Read the model definition and answer for the solid it produces. Units are mm, in the model's axes. Coordinates: 2 decimals unless noted, no trailing zeros. Order: outer loops, then holes, each group sorted by start corner. A loop starts at its lowest first (then second) coordinate and runs counter-clockwise, first axis right, second up. Notation, with made-up numbers: (81.25, -25) -> (138.25, -25) arc R11 ccw to (138.25, -13) -> close; hole circle Ø9 at (89.5, 80.25). An arc over 180 degrees is marked (long way). Return JSON: item names as keys, results as strings. Group by question number.
```python
from build123d import *

# Parameters (mm, degrees)
IZIM1_R                     = 455
Y_KSEKLIK_EKSTR_ZYON1_DEPTH = 12
IZIM2_R                     = 12.5
KES_EKSTR_ZYON1_DEPTH       = 644.579054973
F_8_5_8_5_AP_DELIK1_D       = 8.5


with BuildPart() as part:
    # Çizim1 → Yükseklik-Ekstrüzyon1 (new body)
    with BuildSketch(Plane.XY):
        Circle(IZIM1_R)
    extrude(amount=Y_KSEKLIK_EKSTR_ZYON1_DEPTH)

    # Çizim2 → Kes-Ekstrüzyon1 (cut, through all)
    with BuildSketch(Plane.XY.offset(12)):
        Circle(IZIM2_R)
    extrude(amount=-KES_EKSTR_ZYON1_DEPTH, mode=Mode.SUBTRACT)

    # Ø8.5 (8.5) Çap Delik1 (through all)
    with Locations(Plane.XY.offset(12)):
        with Locations((0, 419), (419, 0), (0, -419), (-419, 0)):
            Hole(F_8_5_8_5_AP_DELIK1_D / 2)


solid = part.part
```
1. Straight lines are drawn through the part: L1, parallel to Y at x = 417, z = 10.5; L2, parallel to X at y = -418, z = 9.5; L3, parallel to Y at x = 419, z = 8.5. For each, find the intervals that lie inside material, in ascending order.
2. Find section C-C on x = -222. Determine the outline of the cut face in (y, z).
3. Find section A-A on z = 3. Determine the outline of the cut face in (x, y), and give its area (3 significant figures).
4. For a pull along Y with two mould halves and no side action, classify faces 1 (the face through (-6, -95, 0)), 2 (the face through (433.99, 136.67, 5.92)), 3 (the face through (11.923, 3.755, 6.084)) as released by +Y, released by -Y, zero draft, split by the parting line, or undercut.
5. Given pin 1 (3 mm diameter, centred on x = 301, z = 4, fed in from +Y); pin 2 (10 mm diameter, centred on x = 0, y = -419, fed in from +Z); pin 3 (2 mm diameter, centred on y = 145.5, z = 5.5, fed in from +X); pin 4 (6 mm diameter, centred on x = 125.5, z = 5, fed in from +Y), each flat-ended and moving along its own axis, determine where each tip first touches the part or whether it passes through.
6. Find section B-B on y = -392. Determine the outline of the cut face in (x, z), and give its area (3 significant figures).
Result:
{
 "1": {"L1": "-182.03 to -3.75, 3.75 to 182.03", "L2": "-179.72 to -4.13, 4.13 to 179.72", "L3": "-177.38 to -4.25, 4.25 to 177.38"},
 "2": {"outline": "(-397.17, 0) -> (397.17, 0) -> (397.17, 12) -> (-397.17, 12) -> close"},
 "3": {"outline": "circle Ø910 at (0, 0); hole circle Ø8.5 at (-419, 0); hole circle Ø25 at (0, 0); hole circle Ø8.5 at (0, -419); hole circle Ø8.5 at (0, 419); hole circle Ø8.5 at (419, 0)", "area": "650,000 mm^2"},
 "4": {"face 1": "zero draft", "face 2": "split by the parting line", "face 3": "undercut"},
 "5": {"pin 1": "y = 342.53", "pin 2": "z = 12", "pin 3": "x = 431.44", "pin 4": "y = 438.2"},
 "6": {"outline": "(-231, 0) -> (231, 0) -> (231, 12) -> (-231, 12) -> close", "area": "5,540 mm^2"}
}
